Read the model definition and answer for the solid it produces. Units are mm, in the model's axes. Coordinates: 2 decimals unless noted, no trailing zeros. Order: outer loops, then holes, each group sorted by start corner. A loop starts at its lowest first (then second) coordinate and runs counter-clockwise, first axis right, second up. Notation, with made-up numbers: (15.5, -21) -> (65.5, -21) arc R18 ccw to (65.5, -16) -> close; hole circle Ø8 at (-34.5, 76). An arc over 180 degrees is marked (long way). Answer as a JSON object with one key per item and string values. Group by question number.
1) Consider L1, parallel to X at y = 23, z = 4.6; L2, parallel to X at y = 10, z = 1.6; L3, parallel to Y at x = -22.5, z = 1.7. Determine where each line is inside the solid, lowest interval first.
2) Section A-A on y = 22 is taken. Determine the outline of the cut face in (x, z).
3) Section B-B on x = -23 is taken. Determine the outline of the cut face in (y, z), and give its area (3 significant figures).
4) Section C-C on x = 50.5 is taken. Determine the outline of the cut face in (y, z), and give its area (3 significant figures).
5) Given pin 1 (1.5 mm diameter, centred on x = 27, z = 3.5, fed in from -Y); pin 2 (1.5 mm diameter, centred on y = -34, z = 3, fed in from +X); pin 3 (1 mm diameter, centred on y = -7.5, z = 1, fed in from +X), each flat-ended and moving along its own axis, determine where each tip first touches the part or whether it passes through.
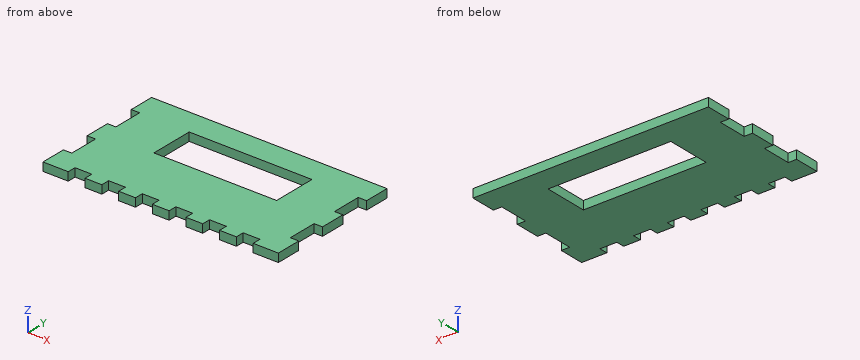
from build123d import *

# Parameters (mm, degrees)
BOSS_EXTRUDE1_DEPTH = 5
SKETCH3_W           = 73
SKETCH3_H           = 26
CUT_EXTRUDE1_DEPTH  = 84.023651357


with BuildPart() as part:
    # Sketch1 → Boss-Extrude1 (new body)
    with BuildSketch(Plane.XY):
        Polygon((69.038630962, -4.683293815), (64.038630962, -4.683293815), (64.038630962, -22.183293815), (69.038630962, -22.183293815), (69.038630962, -37.183293815), (54.044687612, -37.183293815), (54.044687612, -32.183293815), (44.044687612, -32.183293815), (44.044687612, -37.183293815), (34.044687612, -37.183293815), (34.044687612, -32.183293815), (24.044687612, -32.183293815), (24.044687612, -37.183293815), (14.044687612, -37.183293815), (14.044687612, -32.183293815), (4.044687612, -32.183293815), (4.044687612, -37.183293815), (-5.955312388, -37.183293815), (-5.955312388, -32.183293815), (-15.955312388, -32.183293815), (-15.955312388, -37.183293815), (-25.955312388, -37.183293815), (-25.955312388, -32.183293815), (-35.955312388, -32.183293815), (-35.955312388, -37.183293815), (-45.955312388, -37.183293815), (-45.955312388, -32.183293815), (-55.955312388, -32.183293815), (-55.955312388, -37.183293815), (-70.955312388, -37.183293815), (-70.955312388, -22.183293815), (-65.955312388, -22.183293815), (-65.955312388, -4.683293815), (-70.955312388, -4.683293815), (-70.955312388, 10.316706185), (-65.955312388, 10.316706185), (-65.955312388, 27.816706185), (-70.955312388, 27.816706185), (-70.955312388, 42.816706185), (69.044687612, 42.816706185), (69.044687612, 27.816706185), (64.038630962, 27.816706185), (64.038630962, 10.316706185), (69.038630962, 10.316706185), align=None)
    extrude(amount=BOSS_EXTRUDE1_DEPTH)

    # Sketch3 → Cut-Extrude1 (cut, through all)
    with BuildSketch(Plane.XY.offset(5)):
        with Locations((0, 14.816706185)):
            Rectangle(SKETCH3_W, SKETCH3_H)
    extrude(amount=-CUT_EXTRUDE1_DEPTH, mode=Mode.SUBTRACT)


solid = part.part
Worked answers:
{
 "1": {"L1": "x = -65.96 to -36.5, 36.5 to 64.04", "L2": "x = -70.96 to -36.5, 36.5 to 69.04", "L3": "y = -37.18 to 1.82, 27.82 to 42.82"},
 "2": {"outline": "(-65.96, 0) -> (-36.5, 0) -> (-36.5, 5) -> (-65.96, 5) -> close; (36.5, 0) -> (64.04, 0) -> (64.04, 5) -> (36.5, 5) -> close"},
 "3": {"outline": "(-37.18, 0) -> (1.82, 0) -> (1.82, 5) -> (-37.18, 5) -> close; (27.82, 0) -> (42.82, 0) -> (42.82, 5) -> (27.82, 5) -> close", "area": "270 mm²"},
 "4": {"outline": "(-32.18, 0) -> (42.82, 0) -> (42.82, 5) -> (-32.18, 5) -> close", "area": "375 mm²"},
 "5": {"pin 1": "stops at y = -32.18", "pin 2": "stops at x = 69.04", "pin 3": "stops at x = 64.04"}
}
